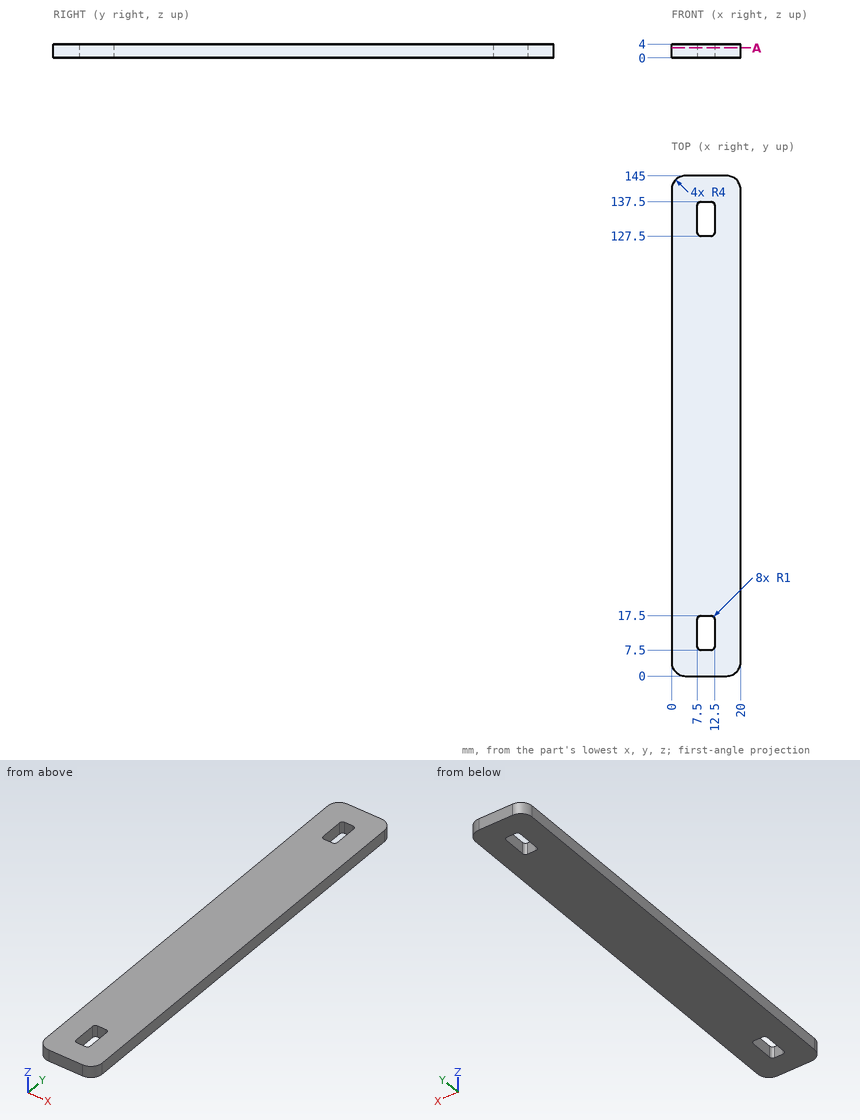
The figure shows three views and two pictorial views of one solid part (mm, origin at its lowest corner). Answer the questions. Give positions to 0.01 mm unless a question says otherwise; leave off trailing zeros. Order: outer loops, then holes, each group sorted by start corner. A loop starts at its lowest first (then second) coordinate and runs counter-clockwise, first axis right, second up. Notation, with made-up numbers: (-24.75, 75) - (25.25, 75) arc R15 ccw to (25.25, 81) - close; hole circle Ø9 at (19.25, 84.5). An arc over 180 degrees is marked (long way). Answer as CSV lines item,"result".
Q1. This flat-tipped pin is pushed along its axis until it touches: pin 1 Ø1.5 at (x, y) = (10.5, 129) entering from +Z. Where does it stop, or does it pass through?
Answer key:
pin 1,"passes through"
Q2. Straight lines are drawn through the part: L1, parallel to Y at x = 10, z = 1.3; L2, parallel to Y at x = 12, z = 3.65; L3, parallel to X at y = 136, z = 0.35. For each, find the intervals that lie inside material, in ascending order.
Answer key:
L1,"y = 0 to 7.5, 17.5 to 127.5, 137.5 to 145"
L2,"y = 0 to 7.63, 17.37 to 127.63, 137.37 to 145"
L3,"x = 0 to 7.5, 12.5 to 20"
Q3. A cutting plane is placed at A-A, the plane z = 2.9. Determine the outline of the cut face in (x, y), and give its area (3 significant figures).
Answer key:
outline,"(0, 4) arc R4 ccw to (4, 0) - (16, 0) arc R4 ccw to (20, 4) - (20, 141) arc R4 ccw to (16, 145) - (4, 145) arc R4 ccw to (0, 141) - close; hole (7.5, 8.5) arc R1 ccw to (8.5, 7.5) - (11.5, 7.5) arc R1 ccw to (12.5, 8.5) - (12.5, 16.5) arc R1 ccw to (11.5, 17.5) - (8.5, 17.5) arc R1 ccw to (7.5, 16.5) - close; hole (7.5, 128.5) arc R1 ccw to (8.5, 127.5) - (11.5, 127.5) arc R1 ccw to (12.5, 128.5) - (12.5, 136.5) arc R1 ccw to (11.5, 137.5) - (8.5, 137.5) arc R1 ccw to (7.5, 136.5) - close"
area,"2,790 mm^2"
